Read the model definition and answer for the solid it produces. Units are mm, in the model's axes. A direction names the side the tool comes from. Coordinates: 2 decimals unless noted, no trailing zeros. Order: outer loops, then holes, each group sorted by start corner. A loop starts at its lowest first (then second) coordinate and runs counter-clockwise, first axis right, second up.
Autodesk Inventor part; units mm, degrees
ref_plane "YZ Plane" through (0, 0, 0) normal (1, 0, 0) x (0, 1, 0)
ref_plane "XZ Plane" through (0, 0, 0) normal (0, 1, 0) x (-1, 0, 0)
ref_plane "XY Plane" through (0, 0, 0) normal (0, 0, 1) x (1, 0, 0)
sketch "Sketch4" plane through (0, 0, 0) normal (0, 0, 1) x (1, 0, 0)
  circle A0 centre (-12.5, 0) radius 0.75
  circle A1 centre (-12.5, 0) radius 1.25
  circle A2 centre (12.5, 0) radius 0.75
  circle A3 centre (12.5, 0) radius 1.25
  line L0 (-12.5, 0.75) -> (12.5, 0.75)
  line L1 (12.5, -0.75) -> (-12.5, -0.75)
  point P0 (0, 0)
  dimension "d22" = 1.5
  dimension "d23" = 2.5
  dimension "d24" = 1.5
  dimension "d25" = 2.5
extrude "Extrusion6" add sketch "Sketch4" along normal mid plane 1.5 contours A0 L0 A1 L1 | A0 L1 A1 L0 | L0 A2 L1 A3 | A3 L1 A2 L0
extrude "Extrusion7" add sketch "Sketch4" along normal mid plane 1 contours A0 L0 A1 L1 | L0 A3 L1 A1 | L0 A2 L1 A3 picked at (-11.4262, -0.0887) picked at (11.582, -0.5653)
properties part number "Shaft_Piston"
1) Determine the mould class of faces 4 (the cylindrical face through (-13.25, 0.03, 0.01)), 5 (the cylindrical face through (13.655, -0.479, 0.01)), 6 (the flat face through (0, 0, -0.5)) for opening direction Y: pulls with the +Y half, pulls with the -Y half, needs draft (parallel to the pull), parting line crosses it, or undercut.
A:
face 4: undercut
face 5: parting line crosses it
face 6: needs draft
2) Straight lines are drawn through the part: line 1 (X direction, y = 0, z = -0.25); line 2 (Y direction, x = -12.5, z = 0.3); line 3 (X direction, y = -0.4, z = -0.6). For each, find the intervals that lie inside material, in ascending order.
A:
line 1: x = -13.75 to -13.25, -11.75 to 11.75, 13.25 to 13.75
line 2: y = -1.25 to -0.75, 0.75 to 1.25
line 3: x = -13.68 to -13.13, -11.87 to -11.32, 11.32 to 11.87, 13.13 to 13.68
3) A cutting plane is placed at D-D, the plane x = -12. Determine the outline of the cut face in (y, z), and give its area (3 significant figures).
A:
outline: (-1.15, -0.75) - (-0.56, -0.75) - (-0.56, 0.75) - (-1.15, 0.75) - close; (0.56, -0.75) - (1.15, -0.75) - (1.15, 0.75) - (0.56, 0.75) - close
area: 1.76 mm2
4) A cutting plane is placed at B-B, the plane y = 0. Determine the outline of the cut face in (x, z).
A:
outline: (-13.75, -0.75) - (-13.25, -0.75) - (-13.25, 0.75) - (-13.75, 0.75) - close; (-11.75, -0.75) - (-11.25, -0.75) - (-11.25, -0.5) - (11.25, -0.5) - (11.25, -0.75) - (11.75, -0.75) - (11.75, 0.75) - (11.25, 0.75) - (11.25, 0.5) - (-11.25, 0.5) - (-11.25, 0.75) - (-11.75, 0.75) - close; (13.25, -0.75) - (13.75, -0.75) - (13.75, 0.75) - (13.25, 0.75) - close
5) Which of the six approach directions +Z, -Z, +X, -X, +Y, -Y give full straight-line access (tool end or side, diameter ignored) to faces 1 (the flat face through (0, 0.75, 0)), 2 (the cylindrical face through (11.75, -0.03, -0.01)), 3 (the flat face through (0, -0.75, 0))?
A:
face 1: +Z, -Z, +Y
face 2: +Z, -Z
face 3: +Z, -Z, -Y
6) A cutting plane is placed at C-C, the plane z = 0.15. Determine the outline of the cut face in (x, y), and give its area (3 significant figures).
A:
outline: (-11.5, -0.75) - (11.5, -0.75) arc R1.25 ccw (long way) to (11.5, 0.75) - (-11.5, 0.75) arc R1.25 ccw (long way) to start; hole circle Ø1.5 at (-12.5, 0); hole circle Ø1.5 at (12.5, 0)
area: 40.3 mm2
7) A cutting plane is placed at A-A, the plane x = 12.5. Determine the outline of the cut face in (y, z).
A:
outline: (-1.25, -0.75) - (-0.75, -0.75) - (-0.75, 0.75) - (-1.25, 0.75) - close; (0.75, -0.75) - (1.25, -0.75) - (1.25, 0.75) - (0.75, 0.75) - close
8) Flat-ended cylindrical pins translate along their axes: pin 1 Ø0.9 at (x, y) = (-12.5, 0) entering from -Z; pin 2 Ø0.8 at (x, z) = (5.5, 0) entering from -Y; pin 3 Ø0.8 at (x, y) = (-1, 0.5) entering from -Z. Find the tip coordinate at first contact, or state that the pin passes through.
A:
pin 1: passes through
pin 2: stops at y = -0.75
pin 3: stops at z = -0.5
